Input: dimensioned drawing with shaded views. Units: mm. Origin: part minimum x, y, z. A direction names the side the tool comes from. Coordinates: 2 decimals unless noted, no trailing zeros. Loops run counter-clockwise (first coordinate to the right, second up) from the corner with the lowest first, then second, coordinate; pieces in that order, holes last.
Item 1: Section query C-C, the plane z = 1.5. Return the cut outline in (x, y), then the cut area to 3 significant figures.
Item 2: Section query B-B, the plane y = 46.5. Return the cut outline in (x, z) (3 decimals), then the cut area to 3 significant figures.
Item 3: Reachability of the marked faces 5, 6, 7 and 8 from +Z, -Z, +X, -X, +Y, -Y: full face, straight path, thin tool, end or side. Return the list, or none.
Item 4: Pin query (flat end, axial travel): pin 1 Ø4 at (y, z) = (87.5, 13.5) entering from -X; pin 2 Ø4 at (x, z) = (30.5, 13.5) entering from +Y; pin 3 Ø4 at (y, z) = (8.5, 11.5) entering from +X. Return the tip coordinate at first contact, or that it passes through.
Item 5: Line query: probe 1 along Y at (x, z) = (84.5, 2.5); probe 2 along Y at (x, z) = (105, 5.5); probe 3 along Y at (x, z) = (116.5, 1). Output: solid intervals per line, ascending.
Item 6: Section query D-D, the plane x = 140. Return the cut outline in (y, z) (3 decimals), then the cut area to 3 significant figures.
Item 7: Section query A-A, the plane x = 80.5. Return the cut outline in (y, z) (3 decimals), then the cut area to 3 significant figures.
Item 8: Pull-direction query (X, two-part tool) for the marked faces 1, 2, 3 and 4; classes: +X half, -X half, draft (parallel to the pull), parting line (faces both ways), or undercut.
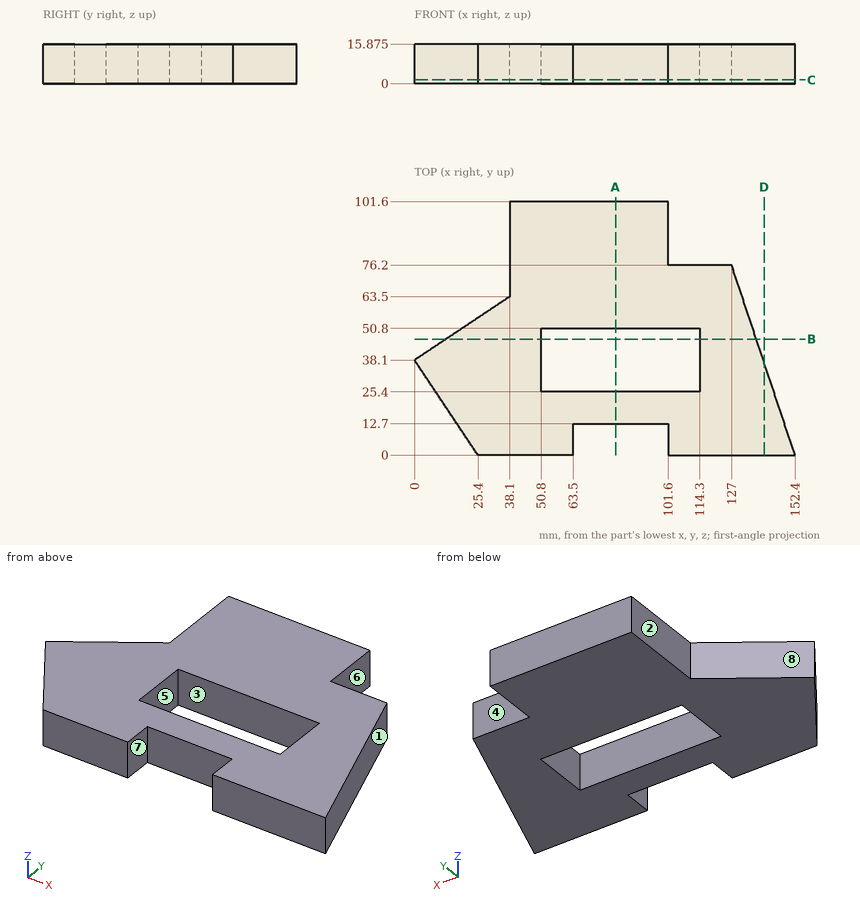
Verdict:
1. outline: (0, 38.1) - (25.4, 0) - (63.5, 0) - (63.5, 12.7) - (101.6, 12.7) - (101.6, 0) - (152.4, 0) - (127, 76.2) - (101.6, 76.2) - (101.6, 101.6) - (38.1, 101.6) - (38.1, 63.5) - close; hole (50.8, 25.4) - (114.3, 25.4) - (114.3, 50.8) - (50.8, 50.8) - close
1. area: 8,710 mm2
2. outline: (12.6, 0) - (50.8, 0) - (50.8, 15.875) - (12.6, 15.875) - close; (114.3, 0) - (136.9, 0) - (136.9, 15.875) - (114.3, 15.875) - close
2. area: 965 mm2
3. face 5: +Z, -Z
3. face 6: +Z, -Z, +X, +Y
3. face 7: +Z, -Z, -Y
3. face 8: +Z, -Z, -X, +Y
4. pin 1: stops at x = 38.1
4. pin 2: stops at y = 59.77
4. pin 3: stops at x = 150.23
5. probe 1: y = 12.7 to 25.4, 50.8 to 101.6
5. probe 2: y = 0 to 25.4, 50.8 to 76.2
5. probe 3: y = 0 to 76.2
6. outline: (0, 0) - (37.2, 0) - (37.2, 15.875) - (0, 15.875) - close
6. area: 591 mm2
7. outline: (12.7, 0) - (25.4, 0) - (25.4, 15.875) - (12.7, 15.875) - close; (50.8, 0) - (101.6, 0) - (101.6, 15.875) - (50.8, 15.875) - close
7. area: 1,010 mm2
8. face 1: +X half
8. face 2: -X half
8. face 3: undercut
8. face 4: draft
